```python
from build123d import *

# Parameters (mm, degrees)
CROQUIS2_W              = 26
CROQUIS2_H              = 2
CORTAR_EXTRUIR1_DEPTH   = 14
CROQUIS3_W              = 27
CROQUIS3_H              = 10
SALIENTE_EXTRUIR1_DEPTH = 24
CORTAR_EXTRUIR2_DEPTH   = 10
CROQUIS5_R              = 1.5
CORTAR_EXTRUIR3_DEPTH   = 24
CROQUIS6_R              = 2.5
CORTAR_EXTRUIR4_DEPTH   = 24


with BuildPart() as part:
    # Croquis1 → Revolución1 (revolve)
    with BuildSketch(Plane.XY):
        Polygon((-89.778094977, -14.637996222), (-78.782252338, -14.637996222), (-78.782252338, -13.637996222), (-85.782252338, -13.637996222), (-85.782252338, 1.235955759), (-87.782252338, 1.235955759), (-88.782252338, -2.637996222), (-88.782252338, -7.637996222), (-87.782252338, -7.637996222), (-87.782252338, -13.637996222), (-89.778094977, -13.637996222), align=None)
    revolve(axis=Axis((-78.782252338, -14.637996222, 0), (0, 1, 0)))

    # Croquis2 → Cortar-Extruir1 (cut)
    with BuildSketch(Plane(origin=(0, 1.235955759, 0), x_dir=(1, 0, 0), z_dir=(0, 1, 0))):
        with Locations((-78.782252338, -5)):
            Rectangle(CROQUIS2_W, CROQUIS2_H)
        with Locations((-78.782252338, 5)):
            Rectangle(CROQUIS2_W, CROQUIS2_H)
    extrude(amount=-CORTAR_EXTRUIR1_DEPTH, mode=Mode.SUBTRACT)

    # Croquis3 → Saliente-Extruir1 (add)
    with BuildSketch(Plane.XZ.offset(14.637996222)):
        with Locations((-78.782252338, 0)):
            Rectangle(CROQUIS3_W, CROQUIS3_H)
    extrude(amount=SALIENTE_EXTRUIR1_DEPTH)

    # Croquis4 → Cortar-Extruir2 (cut)
    with BuildSketch(Plane(origin=(0, 0, -5), x_dir=(-1, 0, 0), z_dir=(0, 0, -1))):
        with BuildLine():
            Line((92.282252338, -38.637996222), (92.282252338, -23.930005944))
            ThreePointArc((92.282252338, -23.930005944), (78.782252338, -37.430005944), (65.282252338, -23.930005944))
            Line((65.282252338, -23.930005944), (65.282252338, -38.637996222))
            Line((65.282252338, -38.637996222), (92.282252338, -38.637996222))
        make_face()
        with BuildLine():
            Line((92.282252338, -14.637996222), (88.575543682, -14.637996222))
            ThreePointArc((88.575543682, -14.637996222), (91.321379763, -18.927978012), (92.282252338, -23.930005944))
            Line((92.282252338, -23.930005944), (92.282252338, -14.637996222))
        make_face()
        with BuildLine():
            Line((65.282252338, -14.637996222), (65.282252338, -23.930005944))
            ThreePointArc((65.282252338, -23.930005944), (66.243124914, -18.927978012), (68.988960995, -14.637996222))
            Line((68.988960995, -14.637996222), (65.282252338, -14.637996222))
        make_face()
        with BuildLine():
            ThreePointArc((71.988960995, -14.637996222), (78.782252338, -35.498695349), (85.575543682, -14.637996222))
            Line((85.575543682, -14.637996222), (71.988960995, -14.637996222))
        make_face()
    extrude(amount=-CORTAR_EXTRUIR2_DEPTH, mode=Mode.SUBTRACT)

    # Croquis5 → Cortar-Extruir3 (cut)
    with BuildSketch(Plane(origin=(0, -13.637996222, 0), x_dir=(1, 0, 0), z_dir=(0, 1, 0))):
        with Locations((-78.782252338, 0)):
            Circle(CROQUIS5_R)
    extrude(amount=-CORTAR_EXTRUIR3_DEPTH, mode=Mode.SUBTRACT)

    # Croquis6 → Cortar-Extruir4 (cut)
    with BuildSketch(Plane.XZ.offset(14.637996222)):
        with Locations((-78.782252338, 0)):
            Circle(CROQUIS6_R)
    extrude(amount=CORTAR_EXTRUIR4_DEPTH, mode=Mode.SUBTRACT)


solid = part.part
```
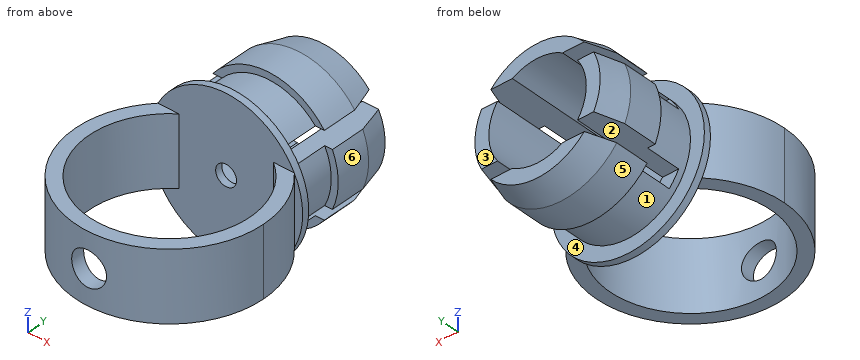
CAD build for the part. Positions are in the model's coordinates, mm. Face numbers are marked on the shaded views. A direction names the side the tool comes from. Round coordinates to 2 decimals unless told otherwise and drop trailing zeros. Write each loop counter-clockwise with the first axis right and the second up, starting at its lowest first coordinate (ties: lowest second). Pieces come first, ordered by that corner, then holes. Notation, with made-up numbers: (37, 20) -> (71, 20) arc R11 ccw to (71, 33) -> close; hole circle Ø2 at (55.5, 55). An arc over 180 degrees is marked (long way). Answer in a Markdown table with one row per item. Add a question column.
Item 1: Mould opens along Y. For the marked faces 1, 2 and 3 say: pulls with the +Y half, pulls with the -Y half, needs draft (parallel to the pull), parting line crosses it, or undercut.
Item 2: Drill centre lines: line 1 (X direction, y = -14.15, z = 0); line 2 (Z direction, x = -71, y = -5.5); line 3 (Z direction, x = -73.75, y = -12.5). Where is each one in solid material? Low to high. Write a range as from..to.
Item 3: Saw through at C-C, the plane y = -29. Write the cut outline in (x, z), then the cut area to 3 significant figures.
Item 4: Drop flat-ended pins along their axis: pin 1 Ø1 at (x, z) = (-68.5, -1.5) entering from -Y; pin 2 Ø2.5 at (x, y) = (-86, -8.5) entering from +Z; pin 3 Ø1.3 at (x, y) = (-85.5, -7) entering from -Z. Give the stop position or say it passes through.
Item 5: Saw through at A-A, the plane y = -17. Write the cut outline in (x, z).
Item 6: Which spindle directions (+Z, -Z, +X, -X, +Y, -Y) get a long thin tool onto all of the face, cutting with end or side? Do the marked faces 4, 5 and 6. Say none if no direction does.
Findings below:
| question | item | result |
|---|---|---|
| 1 | face 1 | undercut |
| 1 | face 2 | needs draft |
| 1 | face 3 | pulls with the +Y half |
| 2 | line 1 | x = -89.78..-80.28, -77.28..-67.79 |
| 2 | line 2 | z = -6.28..-6, -4..4, 6..6.28 |
| 2 | line 3 | z = -7.46..-6, 6..7.46 |
| 3 | outline | (-91.29, -5) -> (-89.16, -5) -> (-89.16, 5) -> (-91.29, 5) -> close; (-68.4, -5) -> (-66.27, -5) -> (-66.27, 5) -> (-68.4, 5) -> close |
| 3 | area | 42.7 mm^2 |
| 4 | pin 1 | stops at y = -33.23 |
| 4 | pin 2 | stops at z = 7.76 |
| 4 | pin 3 | stops at z = -7.95 |
| 5 | outline | (-90.37, -5) -> (-87.98, -5) -> (-87.98, 5) -> (-90.37, 5) -> close; (-69.58, -5) -> (-67.2, -5) -> (-67.2, 5) -> (-69.58, 5) -> close |
| 6 | face 4 | none |
| 6 | face 5 | -Z, +Y |
| 6 | face 6 | +X, +Y |
